Answer from the drawing. Dimensions are ordinates in mm from the lowest x, y and z of the part. A direction names the side the tool comes from. Round coordinates to 2 decimals unless told otherwise and drop trailing zeros. Write each loop counter-clockwise with the first axis right and the second up, starting at its lowest first coordinate (ties: lowest second). Pieces come first, ordered by that corner, then holes. Notation, with made-up numbers: (-28.5, 29) - (20.5, 29) arc R20 ccw to (20.5, 40) - close; hole circle Ø7 at (48, 60.25). An arc over 180 degrees is marked (long way). Answer as a JSON object with one key per item and string values.
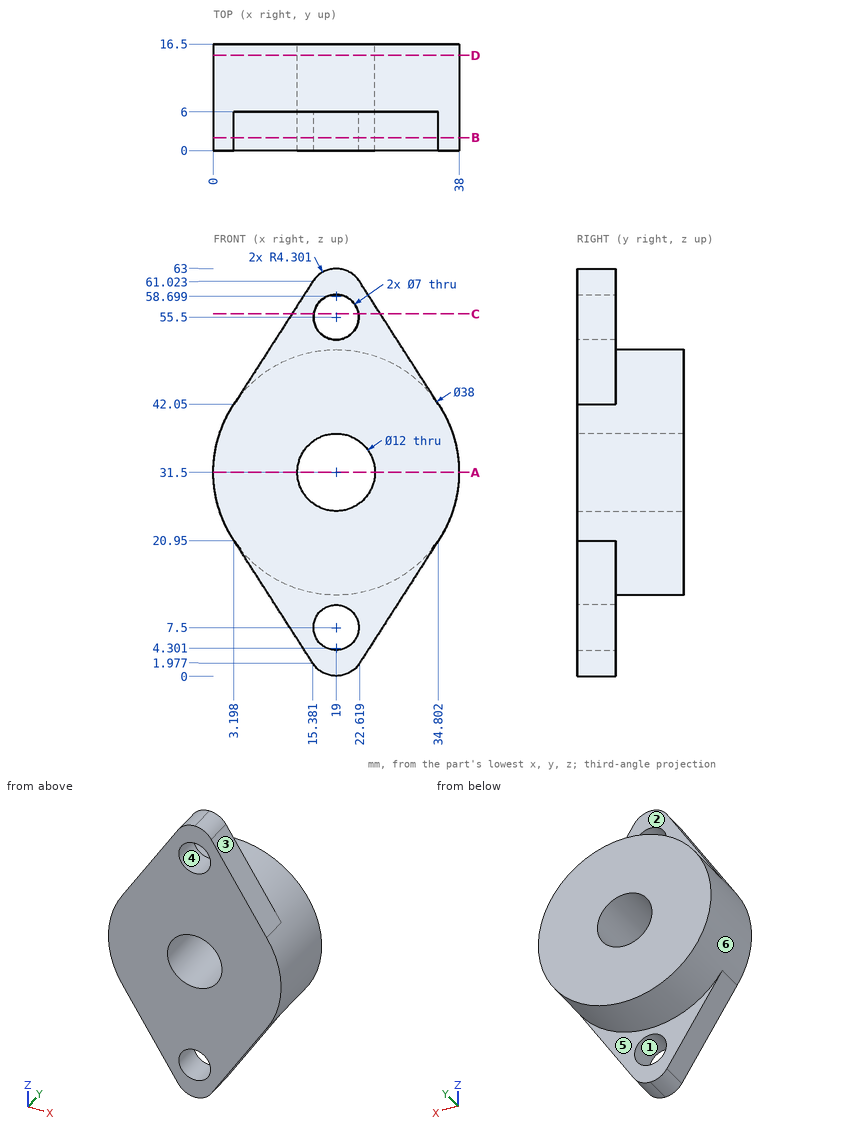
Item 1: Each of these flat-tipped pins is pushed along its axis until it touches: P1, Ø17, axis at x = 13, z = 56, coming from the +Y side; P2, Ø1.5, axis at y = 13, z = 14.5, coming from the +X side (1 decimal); P3, Ø8, axis at y = 13, z = 55, coming from the -X side; P4, Ø1, axis at x = 21, y = 7, coming from the +Z side. Where does it stop, or does it pass through?
Results found:
{"P1": "y = 16.5", "P2": "x = 28.8", "P3": "through", "P4": "z = 50.44"}
Item 2: Determine the mould class of the marked faces 1, 2 and 3 for opening direction Z: pulls with the +Z half, pulls with the -Z half, needs draft (parallel to the pull), parting line crosses it, or undercut.
Results found:
{"face 1": "undercut", "face 2": "needs draft", "face 3": "pulls with the +Z half"}
Item 3: Consider line 1 along X through (y, z) = (4, 31.5); line 2 along Z through (x, y) = (24, 7) (1 decimal); line 3 along Z through (x, y) = (22, 3.5) (1 decimal). Determine where each line is inside the solid, lowest interval first.
Results found:
{"line 1": "0 to 13, 25 to 38", "line 2": "13.2 to 28.2, 34.8 to 49.8", "line 3": "1.2 to 5.7, 9.3 to 26.3, 36.7 to 53.7, 57.3 to 61.8"}
Item 4: A cutting plane is placed at D-D (y = 14.75). Write down the section's boundary in (x, z).
Results found:
{"outline": "circle Ø38 at (19, 31.5); hole circle Ø12 at (19, 31.5)"}
Item 5: A cutting plane is placed at B-B (y = 2). Write down the section's boundary in (x, z), and give its area (3 significant figures).
Results found:
{"outline": "(3.2, 20.95) - (15.38, 1.98) arc R4.3 ccw to (22.62, 1.98) - (34.8, 20.95) arc R19 ccw to (34.8, 42.05) - (22.62, 61.02) arc R4.3 ccw to (15.38, 61.02) - (3.2, 42.05) arc R19 ccw to start; hole circle Ø12 at (19, 31.5); hole circle Ø7 at (19, 7.5); hole circle Ø7 at (19, 55.5)", "area": "1,330 mm²"}
Item 6: A cutting plane is placed at A-A (z = 31.5). Write down the section's boundary in (x, y).
Results found:
{"outline": "(0, 0) - (13, 0) - (13, 16.5) - (0, 16.5) - close; (25, 0) - (38, 0) - (38, 16.5) - (25, 16.5) - close"}
Item 7: For the marked faces 4, 5 and 6, determine the directions among +Z, -Z, +X, -X, +Y, -Y from which every point of the face is accessible in a straight line to the end or side of a thin tool.
Results found:
{"face 4": "+Y, -Y", "face 5": "-Z, +Y", "face 6": "+Y"}
Item 8: A cutting plane is placed at C-C (z = 56). Write down the section's boundary in (x, y) (1 decimal).
Results found:
{"outline": "(12.2, 0) - (15.5, 0) - (15.5, 6) - (12.2, 6) - close; (22.5, 0) - (25.8, 0) - (25.8, 6) - (22.5, 6) - close"}
